Geometry check sheet. Reference: the model listing, model coordinates, mm. A direction names the side the tool comes from. Coordinates: 2 decimals unless noted, no trailing zeros. Order: outer loops, then holes, each group sorted by start corner. A loop starts at its lowest first (then second) coordinate and runs counter-clockwise, first axis right, second up. Notation, with made-up numbers: (-29.5, 47.5) - (-0.5, 47.5) arc R23 ccw to (-0.5, 55.5) - close; hole circle Ø4 at (53.5, 71.5). An arc over 180 degrees is marked (long way). Return JSON: item names as keys, results as strings. Group by question number.
Item 1: Section check A-A on x = -2.5. Enter the section's corners in (y, z).
Item 2: Tool access check on faces 1 (the flat face through (-17.5, 7, 4)), 2 (the flat face through (-25, 7, 8)), 3 (the flat face through (39.5, 42, -10)). Record the directions out of +Z, -Z, +X, -X, +Y, -Y that give a thin tool (end or side, any length) a straight path to the whole face; none if there is none.
Item 3: Section check D-D on y = 13. Enter the section's corners in (x, z).
Item 4: Section check B-B on z = 6. Enter the section's corners in (x, y), then the cut area to 3 significant figures.
Item 5: Draft check along Z on faces 4 (the flat face through (44, 27, 0)), 5 (the flat face through (-2, 7, -8)), 6 (the flat face through (59.5, 35, -10)), 7 (the flat face through (-14, 11, -20)). Enter one of: pulls with the +Z half, pulls with the -Z half, needs draft (parallel to the pull), parting line crosses it, or undercut.
Item 6: Gauge pin test, flat ends, axial feed: pin 1 (16.5 mm diameter, centred on x = -1.5, y = 11, fed in from +Z); pin 2 (12 mm diameter, centred on x = 45.5, y = 25.5, fed in from +Z); pin 3 (4.5 mm diameter, centred on y = 11, z = 10.5, fed in from +X); pin 4 (1.5 mm diameter, centred on y = 17, z = 21.5, fed in from -X). Record the tip position at first contact, or that the pin passes through.
Item 7: Scan lines: probe 1 along X at (y, z) = (67, -16); probe 2 along X at (y, z) = (14.5, 16.5); probe 3 along Z at (x, y) = (-2, 8). Record each from-to range of solid material in increasing order.
Item 8: Section check C-C on z = -15. Enter the section's corners in (x, y), then the cut area to 4 significant figures.
Autodesk Inventor part; units mm, degrees
ref_plane "YZ Plane" through (0, 0, 0) normal (1, 0, 0) x (0, 1, 0)
ref_plane "XZ Plane" through (0, 0, 0) normal (0, 1, 0) x (-1, 0, 0)
ref_plane "XY Plane" through (0, 0, 0) normal (0, 0, 1) x (1, 0, 0)
sketch "스케치1" plane through (0, 0, 0) normal (0, 1, 0) x (-1, 0, 0)
  arc A0 (25, 17) -> (-20, 17) centre (2.5, 17) ccw
  arc A1 (17.5, 17) -> (-12.5, 17) centre (2.5, 17) ccw
  line L0 (17.5, 17) -> (-12.5, 17)
  line L1 (-20, 17) -> (-20, 0)
  line L2 (-20, -20) -> (25, -20)
  line L3 (25, 0) -> (25, 17)
  line L4 (-12.5, 17) -> (17.5, 17)
  line L5 (17.5, 17) -> (17.5, 0)
  line L6 (17.5, 0) -> (-12.5, 0)
  line L7 (-12.5, 0) -> (-12.5, 17)
  line L8 (59.5, -20) -> (-59.5, -20)
  line L9 (-59.5, -20) -> (-59.5, 0)
  line L10 (59.5, 0) -> (59.5, -20)
  line L11 (25, 0) -> (59.5, 0)
  line L12 (-59.5, 0) -> (-20, 0)
  line L13 (-12.5, 0) -> (17.5, 0)
  line L14 (17.5, 0) -> (-12.5, 0)
  line L15 (-12.5, 0) -> (-12.5, -8)
  line L16 (-12.5, -8) -> (17.5, -8)
  line L17 (17.5, -8) -> (17.5, 0)
  point P0 (0, 0)
  point P1 (0, 17)
  point P2 (-59.5, -10)
  dimension "d1" = 30
  dimension "d2" = 45
  dimension "d3" = 0
  dimension "d4" = 17
  dimension "d5" = 37
  dimension "d6" = 119
  dimension "d10" = 20
  dimension "d11" = 22.5
  dimension "d12" = 0
  dimension "d13" = 59.5
  dimension "d14" = 8
  dimension "d15" = 39.5
extrude "돌출1" add sketch "스케치1" along normal blind 15
sketch "스케치2" plane through (0, 15, 0) normal (0, 1, 0) x (1, 0, 0)
  point P0 (0, 0)
sketch "스케치3" plane through (0, 15, 0) normal (0, 1, 0) x (1, 0, 0)
  line L0 (-39.5, 0) -> (-59.5, 0)
  line L1 (-59.5, 0) -> (-59.5, 20)
  line L2 (-59.5, 20) -> (-39.5, 20)
  line L3 (-39.5, 20) -> (-39.5, 0)
  line L4 (-39.5, 0) -> (-59.5, 20) construction
  line L5 (-59.5, 0) -> (-39.5, 20) construction
  line L6 (-59.5, 20) -> (-59.5, 0)
  line L7 (-59.5, 0) -> (-25, 0)
  line L8 (0, 0) -> (0, 5.3551)
  line L9 (39.5, 0) -> (59.5, 0)
  line L10 (59.5, 0) -> (59.5, 20)
  line L11 (59.5, 20) -> (39.5, 20)
  line L12 (39.5, 20) -> (39.5, 0)
  line L13 (39.5, 0) -> (59.5, 20) construction
  line L14 (59.5, 0) -> (39.5, 20) construction
  line L15 (59.5, 20) -> (59.5, 0)
  line L16 (59.5, 0) -> (25, 0)
  point P0 (-49.5, 10)
  point P1 (-49.5, 0)
  point P2 (49.5, 10)
  point P3 (49.5, 0)
  dimension "d16" = 20
  dimension "d17" = 20
  dimension "d18" = 0
  dimension "d19" = 0
extrude "돌출2" add sketch "스케치3" along normal blind 55.5
properties part number "액추에이터 지지대 3D 프린트"
Computed:
{
 "1": {"outline": "(0, -20) - (15, -20) - (15, -8) - (0, -8) - close; (0, 32) - (15, 32) - (15, 39.5) - (0, 39.5) - close"},
 "2": {"face 1": "+Y, -Y", "face 2": "+Z, -X, +Y, -Y", "face 3": "+Z, -Z, +Y"},
 "3": {"outline": "(-59.5, -20) - (59.5, -20) - (59.5, 0) - (20, 0) - (20, 17) arc R22.5 ccw to (-25, 17) - (-25, 0) - (-59.5, 0) - close; hole (-17.5, -8) - (12.5, -8) - (12.5, 17) arc R15 ccw to (-17.5, 17) - close"},
 "4": {"outline": "(-25, 0) - (-17.5, 0) - (-17.5, 15) - (-25, 15) - close; (12.5, 0) - (20, 0) - (20, 15) - (12.5, 15) - close", "area": "225 mm²"},
 "5": {"face 4": "pulls with the +Z half", "face 5": "undercut", "face 6": "needs draft", "face 7": "pulls with the -Z half"},
 "6": {"pin 1": "stops at z = 39.5", "pin 2": "stops at z = 0", "pin 3": "stops at x = 20", "pin 4": "passes through"},
 "7": {"probe 1": "x = -59.5 to -39.5, 39.5 to 59.5", "probe 2": "x = -25 to -17.5, 12.5 to 20", "probe 3": "z = -20 to -8, 31.99 to 39.49"},
 "8": {"outline": "(-59.5, 0) - (59.5, 0) - (59.5, 70.5) - (39.5, 70.5) - (39.5, 15) - (-39.5, 15) - (-39.5, 70.5) - (-59.5, 70.5) - close", "area": "4,005 mm²"}
}
